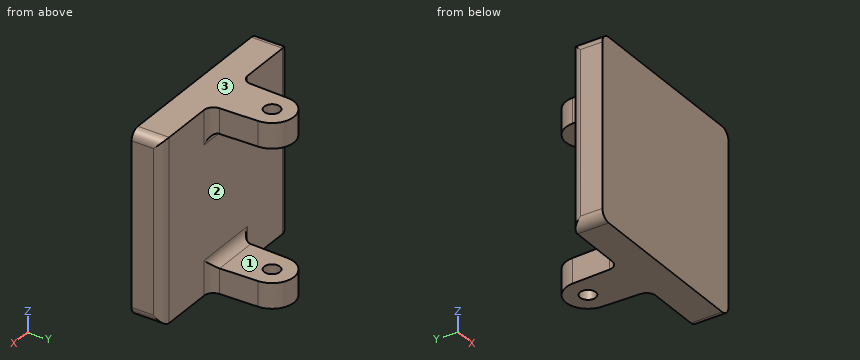
from build123d import *

# Parameters (mm, degrees)
SKETCH2_W           = 60
SKETCH2_H           = 58
BOSS_EXTRUDE1_DEPTH = 10
SKETCH3_R           = 2.5
BOSS_EXTRUDE2_DEPTH = 8
FILLET1_R           = 3


with BuildPart() as part:
    # Sketch2 → Boss-Extrude1 (new body)
    with BuildSketch(Plane(origin=(0, 0, 0), x_dir=(1, 0, 0), z_dir=(0, 1, 0))):
        Rectangle(SKETCH2_W, SKETCH2_H)
    extrude(amount=BOSS_EXTRUDE1_DEPTH)

    # Sketch3 → Boss-Extrude2 (add)
    with BuildSketch(Plane.XY.offset(29)):
        with BuildLine():
            Line((-7.5, 10), (-6.996052809, 25))
            ThreePointArc((-6.996052809, 25), (0, 31.764957256), (6.996052809, 25))
            Line((6.996052809, 25), (7.5, 10))
            Line((7.5, 10), (-7.5, 10))
        make_face()
        with Locations((0, 24.764957256)):
            Circle(SKETCH3_R, mode=Mode.SUBTRACT)
    boss_extrude2 = extrude(amount=-BOSS_EXTRUDE2_DEPTH)

    # Mirror1: Boss-Extrude2 across plane
    add(boss_extrude2.mirror(Plane.XY))

    # Fillet1
    fillet1_edges = [part.edges().sort_by_distance(p)[0] for p in [
        (-30, 10, 0),
        (0, 10, 21),
        (7.5, 10, 25),
        (-7.5, 10, 25),
        (0, 10, -21),
        (-7.5, 10, -25),
        (7.5, 10, -25),
        (30, 10, 0),
        (30, 5, 29),
        (-30, 5, 29),
        (-30, 5, -29),
        (30, 5, -29),
    ]]
    fillet(fillet1_edges, radius=FILLET1_R)


solid = part.part
Here's how the part is built. I have some questions about the finished solid (model axes, mm). Face numbers are marked on the shaded views. A direction names the side the tool comes from. Coordinates: 2 decimals unless noted, no trailing zeros. Order: outer loops, then holes, each group sorted by start corner. A loop starts at its lowest first (then second) coordinate and runs counter-clockwise, first axis right, second up. Notation, with made-up numbers: (-32.5, 82) - (10.5, 82) arc R25 ccw to (10.5, 94) - close; hole circle Ø6 at (-26.75, -19). An arc over 180 degrees is marked (long way). Use CSV: the item, a comma, the result in double quotes. Start each with the question number.
1. Please list where these lines run through material, in increasing order: line 1 (Y direction, x = 0, z = 23.5); line 2 (Z direction, x = -1.5, y = 30); line 3 (Y direction, x = -23, z = -11). Write a range as from..to.
2. Suppose I cut it at D-D on x = -9. List the corners of the cut face in (y, z) for me.
3. Suppose I cut it at A-A on x = 0. List the corners of the cut face in (y, z) for me.
4. Suppose I cut it at B-B on z = -23. List the corners of the cut face in (x, y) for me.
5. Suppose I cut it at C-C on y = 11. List the corners of the cut face in (x, z) for me, then the cut area to 3 significant figures.
6. For the marked faces 1, 2 and 3, which set-ups out of +Z, -Z, +X, -X, +Y, -Y let a thin tool reach every point of the face, with its end or its side?
7. I'm going to push flat-ended pins straight in: pin 1 (3 mm diameter, centred on x = 8, z = 9.5, fed in from +Y); pin 2 (12 mm diameter, centred on x = 5.5, z = 0.5, fed in from -Y); pin 3 (6 mm diameter, centred on y = 20, z = 21.5, fed in from -X). Where does each tip first touch, or does it pass through?
Output:
1,line 1,"y = 0..22.26, 27.26..31.76"
1,line 2,"z = -29..-21, 21..29"
1,line 3,"y = 0..10"
2,outline,"(0, -29) - (10.35, -29) - (10.35, -19.4) arc R3 cw to (10, -18) - (10, 18) arc R3 cw to (10.35, 19.4) - (10.35, 29) - (0, 29) - close"
3,outline,"(0, -29) - (22.26, -29) - (22.26, -21) - (13, -21) arc R3 cw to (10, -18) - (10, 18) arc R3 cw to (13, 21) - (22.26, 21) - (22.26, 29) - (0, 29) - close; (27.26, -29) - (31.76, -29) - (31.76, -21) - (27.26, -21) - close; (27.26, 21) - (31.76, 21) - (31.76, 29) - (27.26, 29) - close"
4,outline,"(-30, 0) - (30, 0) - (30, 7) arc R3 ccw to (27, 10) - (10.4, 10) arc R3 cw to (7.4, 12.9) - (7, 25) arc R7 ccw to (-7, 25) - (-7.4, 12.9) arc R3 cw to (-10.4, 10) - (-27, 10) arc R3 ccw to (-30, 7) - close; hole circle Ø5 at (0, 24.76)"
5,outline,"(-8.16, -29) - (8.16, -29) - (8.16, -20.24) - (-8.16, -20.24) - close; (-8.16, 20.24) - (8.16, 20.24) - (8.16, 29) - (-8.16, 29) - close"
5,area,"286 mm2"
6,face 1,"+X, -X, +Y"
6,face 2,"+Y"
6,face 3,"+Z, +X, -X, +Y, -Y"
7,pin 1,"stops at y = 10"
7,pin 2,"stops at y = 0"
7,pin 3,"stops at x = -7.26"
